Input: dimensioned drawing with shaded views. Units: mm. Origin: part minimum x, y, z. A direction names the side the tool comes from. Give positions to 0.01 mm unless a question says otherwise; leave off trailing zeros. Write each loop counter-clockwise with the first axis right and the second up, starting at its lowest first coordinate (ties: lowest second). Pieces come first, ordered by that corner, then holes.
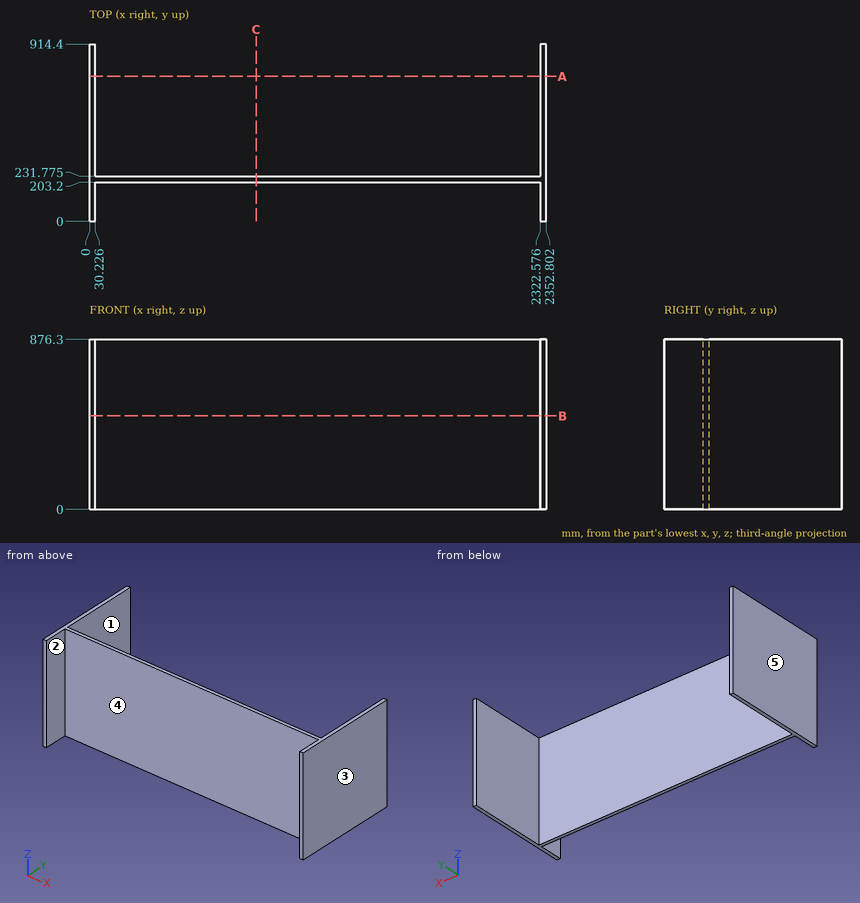
1. Cut plane B-B, the plane z = 482.5. Return the cut outline in (x, y) (3 decimals), then the cut area to 3 significant figures.
2. Contact query for a flat-ended pin moving along its axis: P1, Ø5, axis at x = 487, z = 538.5, coming from the +Y side (3 decimals). Output: stop coordinate, or through.
3. Cut plane C-C, the plane x = 859. Return the cut outline in (y, z) (3 decimals).
4. Access query for the marked faces 1 and 2. Directions: +Z, -Z, +X, -X, +Y, -Y. A direction counts if a zero-diameter tool reaches every point of the face in a straight line with its end or side. Return the directions, or none.
5. Cut plane A-A, the plane y = 747.5. Return the cut outline in (x, z), then the cut area to 3 significant figures.
6. Mould query, pull axis X, two halves, no side actions, for the marked faces 3, 4 and 5. Classes: +X half, -X half, draft (parallel to the pull), parting line (faces both ways), or undercut.
7. Line query: L1, parallel to X at y = 545, z = 488.5; L2, parallel to Y at x = 209, z = 791 (3 decimals). Output: solid intervals per line, ascending.
Response values:
1. outline: (0, 0) - (30.226, 0) - (30.226, 203.2) - (2322.576, 203.2) - (2322.576, 0) - (2352.802, 0) - (2352.802, 914.4) - (2322.576, 914.4) - (2322.576, 231.775) - (30.226, 231.775) - (30.226, 914.4) - (0, 914.4) - close
1. area: 121,000 mm2
2. P1: stops at y = 231.775
3. outline: (203.2, 0) - (231.775, 0) - (231.775, 876.3) - (203.2, 876.3) - close
4. face 1: +Z, -Z, +Y
4. face 2: +Z, -Z, -Y
5. outline: (0, 0) - (30.23, 0) - (30.23, 876.3) - (0, 876.3) - close; (2322.58, 0) - (2352.8, 0) - (2352.8, 876.3) - (2322.58, 876.3) - close
5. area: 53,000 mm2
6. face 3: +X half
6. face 4: undercut
6. face 5: -X half
7. L1: x = 0 to 30.23, 2322.58 to 2352.8
7. L2: y = 203.2 to 231.775
